The model under review builds one solid part; all positions refer to its coordinate system, in mm. A direction names the side the tool comes from. Coordinates: 2 decimals unless noted, no trailing zeros. Loops run counter-clockwise (first coordinate to the right, second up) from the corner with the lowest first, then second, coordinate; pieces in that order, holes last. Notation, with made-up numbers: (-5, -9) - (9, -9) arc R34 ccw to (9, 25) - close; hole circle Ø7 at (79.5, 75). An arc over 180 degrees is marked (long way). One line per item, written item: value. Start each with the question number.
1. For faces 1 (the face through (-5, 8.8, -3)), 2 (the face through (-1.08, 2.12, -4.88)), list the 3-axis set-ups (+Z, -Z, +X, -X, +Y, -Y) from which the entire face can be reached by the end or side of a thin tool; tool diameter is ignored.
2. We need section A-A, the plane z = 0. Give the boundary of the cut face in (x, y) (3 decimals), then the cut area to 3 significant figures.
3. To check wall thickness, follow line 1 (Z direction, x = 0, y = 7) (3 decimals); line 2 (Y direction, x = -2.25, z = 6); line 3 (X direction, y = 6.5, z = 1.25). State the ranges of each line that lie inside material, in increasing order.
4. Insertion check: P1, Ø5, axis at x = 3, y = 6, coming from the +Z side; P2, Ø4, axis at y = 8, z = -3.5, coming from the +X side; P3, Ø5, axis at x = 1.5, z = -1, coming from the -Y side. Each pin has a flat end and moves straight along its axis. Give the tip position at first contact, or say it passes through.
5. We need section D-D, the plane y = 1.25. Give the boundary of the cut face in (x, z) (3 decimals), then the cut area to 3 significant figures.
6. We need section C-C, the plane y = 4.5. Give the boundary of the cut face in (x, z) (3 decimals), then the cut area to 3 significant figures.
7. We need section B-B, the plane x = 0. Give the boundary of the cut face in (y, z) (3 decimals), then the cut area to 3 significant figures.
8. Mouldability with a two-part tool opening along Z and no side actions: class faces 3 (the face through (-5, 0, -3)), 4 (the face through (-1.651, 4.36, 7.434)), 5 (the face through (-1.08, 6.68, 4.88)) as +Z half, -Z half, draft (parallel to the pull), parting line (faces both ways), or undercut.
from build123d import *

# Parameters (mm, degrees)
SKETCH1_R           = 7.615
SKETCH1_R_2         = 4
BOSS_EXTRUDE1_DEPTH = 8.8
SKETCH2_R           = 5
CUT_EXTRUDE1_DEPTH  = 4
SKETCH3_R           = 5
CUT_EXTRUDE2_DEPTH  = 4
CHAMFER1_SIZE       = 0.3
CHAMFER2_SIZE       = 1.51


with BuildPart() as part:
    # Sketch1 → Boss-Extrude1 (new body)
    with BuildSketch(Plane(origin=(0, 0, 0), x_dir=(1, 0, 0), z_dir=(0, 1, 0))):
        Circle(SKETCH1_R)
        Circle(SKETCH1_R_2, mode=Mode.SUBTRACT)
    extrude(amount=BOSS_EXTRUDE1_DEPTH)

    # Sketch2 → Cut-Extrude1 (cut)
    with BuildSketch(Plane(origin=(0, 8.8, 0), x_dir=(1, 0, 0), z_dir=(0, 1, 0))):
        Circle(SKETCH2_R)
    extrude(amount=-CUT_EXTRUDE1_DEPTH, mode=Mode.SUBTRACT)

    # Sketch3 → Cut-Extrude2 (cut)
    with BuildSketch(Plane.XZ):
        Circle(SKETCH3_R)
    extrude(amount=-CUT_EXTRUDE2_DEPTH, mode=Mode.SUBTRACT)

    # Chamfer1
    chamfer1_edges = [part.edges().sort_by_distance(p)[0] for p in [
        (-5, 8.8, 0),
        (-5, 0, 0),
    ]]
    chamfer(chamfer1_edges, length=CHAMFER1_SIZE)

    # Chamfer2
    chamfer2_edges = [part.edges().sort_by_distance(p)[0] for p in [
        (-7.615, 0, 0),
        (-7.615, 8.8, 0),
    ]]
    chamfer(chamfer2_edges, length=CHAMFER2_SIZE)


solid = part.part
Findings below:
1. face 1: +Z, -Z, +X, -X, +Y
1. face 2: -Y
2. outline: (-7.615, 1.51) - (-6.105, 0) - (-5.3, 0) - (-5, 0.3) - (-5, 4) - (-4, 4) - (-4, 4.8) - (-5, 4.8) - (-5, 8.5) - (-5.3, 8.8) - (-6.105, 8.8) - (-7.615, 7.29) - close; (4, 4) - (5, 4) - (5, 0.3) - (5.3, 0) - (6.105, 0) - (7.615, 1.51) - (7.615, 7.29) - (6.105, 8.8) - (5.3, 8.8) - (5, 8.5) - (5, 4.8) - (4, 4.8) - close
2. area: 42.9 mm2
3. line 1: -7.615 to -5, 5 to 7.615
3. line 2: 0.3 to 8.5
3. line 3: -7.51 to -4.84, 4.84 to 7.51
4. P1: z = 7.6
4. P2: x = 7.44
4. P3: y = 4
5. outline: circle Ø14.71 at (0, 0); hole circle Ø10 at (0, 0)
5. area: 91.4 mm2
6. outline: circle Ø15.23 at (0, 0); hole circle Ø8 at (0, 0)
6. area: 132 mm2
7. outline: (0, -6.105) - (1.51, -7.615) - (7.29, -7.615) - (8.8, -6.105) - (8.8, -5.3) - (8.5, -5) - (4.8, -5) - (4.8, -4) - (4, -4) - (4, -5) - (0.3, -5) - (0, -5.3) - close; (0, 5.3) - (0.3, 5) - (4, 5) - (4, 4) - (4.8, 4) - (4.8, 5) - (8.5, 5) - (8.8, 5.3) - (8.8, 6.105) - (7.29, 7.615) - (1.51, 7.615) - (0, 6.105) - close
7. area: 42.9 mm2
8. face 3: draft
8. face 4: parting line
8. face 5: undercut
